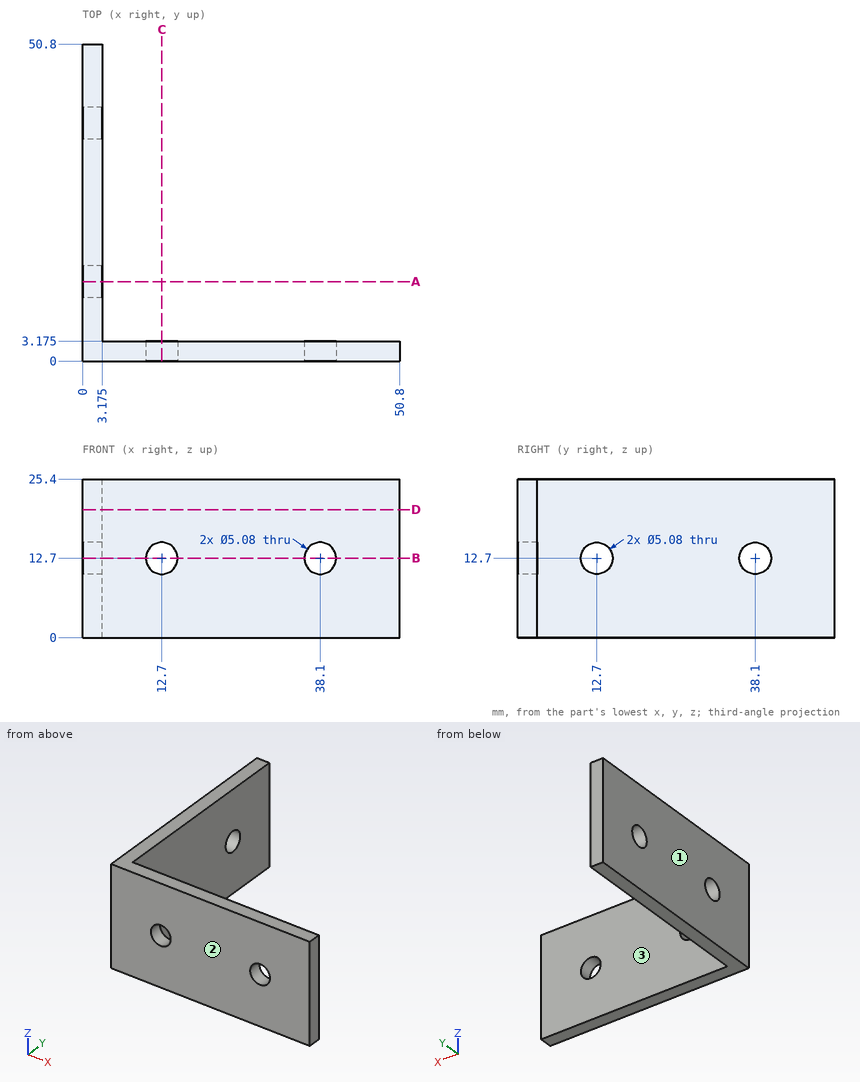
Job drawing, mm, ordinate dimensions from the low corner. One solid piece. Coordinates: 2 decimals unless noted, no trailing zeros. Write each loop counter-clockwise with the first axis right and the second up, starting at its lowest first coordinate (ties: lowest second). Pieces come first, ordered by that corner, then holes.
Item 1: Slice it at D-D (z = 20.5). Write the cut outline in (x, y) (3 decimals).
Item 2: Slice it at B-B (z = 12.7). Write the cut outline in (x, y) (3 decimals).
Item 3: Slice it at A-A (y = 12.7). Write the cut outline in (x, z) (3 decimals), and give its area (3 significant figures).
Item 4: Pin check, flat tips, straight feed: pin 1 (10 mm diameter, centred on x = 13.5, z = 3, fed in from -Y); pin 2 (6 mm diameter, centred on y = 12.7, z = 12.7, fed in from +X) (3 decimals); pin 3 (4.5 mm diameter, centred on x = 38.1, z = 12.7, fed in from -Y). Stop position of each tip, or through.
Item 5: Mould opens along Y. For the marked faces 1, 2 and 3 say: released by +Y, released by -Y, zero draft, split by the parting line, or undercut.
Item 6: Probe line 1 (Y direction, x = 1.85, z = 12.7); line 2 (Z direction, x = 0.85, y = 12.7). List the from-to ranges inside material, lowest first.
Results found:
1. outline: (0, 0) - (50.8, 0) - (50.8, 3.175) - (3.175, 3.175) - (3.175, 50.8) - (0, 50.8) - close
2. outline: (0, 0) - (10.16, 0) - (10.16, 3.175) - (3.175, 3.175) - (3.175, 10.16) - (0, 10.16) - close; (0, 15.24) - (3.175, 15.24) - (3.175, 35.56) - (0, 35.56) - close; (0, 40.64) - (3.175, 40.64) - (3.175, 50.8) - (0, 50.8) - close; (15.24, 0) - (35.56, 0) - (35.56, 3.175) - (15.24, 3.175) - close; (40.64, 0) - (50.8, 0) - (50.8, 3.175) - (40.64, 3.175) - close
3. outline: (0, 0) - (3.175, 0) - (3.175, 10.16) - (0, 10.16) - close; (0, 15.24) - (3.175, 15.24) - (3.175, 25.4) - (0, 25.4) - close
3. area: 64.5 mm2
4. pin 1: stops at y = 0
4. pin 2: stops at x = 3.175
4. pin 3: passes through
5. face 1: zero draft
5. face 2: released by -Y
5. face 3: released by +Y
6. line 1: y = 0 to 10.16, 15.24 to 35.56, 40.64 to 50.8
6. line 2: z = 0 to 10.16, 15.24 to 25.4
